Geometry check sheet. Reference: the model listing, model coordinates, mm. Round coordinates to 2 decimals unless told otherwise and drop trailing zeros. Write each loop counter-clockwise with the first axis right and the second up, starting at its lowest first coordinate (ties: lowest second). Pieces come first, ordered by that corner, then holes. Notation, with made-up numbers: (-12.5, -14) - (39.5, -14) arc R28 ccw to (39.5, 15) - close; hole circle Ø8 at (-8.5, -9). An arc over 180 degrees is marked (long way). Return JSON: item names as keys, results as strings. Group by question number.
from build123d import *

# Parameters (mm, degrees)
CROQUIS1_W              = 60
CROQUIS1_H              = 6
SALIENTE_EXTRUIR1_DEPTH = 3
REDONDEO1_R             = 1
CROQUIS2_R              = 1.5
CROQUIS2_R_2            = 1
CORTAR_EXTRUIR1_DEPTH   = 31.298514815


with BuildPart() as part:
    # Croquis1 → Saliente-Extruir1 (new body)
    with BuildSketch(Plane.XY):
        Rectangle(CROQUIS1_W, CROQUIS1_H)
    extrude(amount=SALIENTE_EXTRUIR1_DEPTH)

    # Redondeo1
    redondeo1_edges = [part.edges().sort_by_distance(p)[0] for p in [
        (30, 0, 3),
        (0, 3, 3),
        (-30, 0, 3),
        (0, 3, 0),
        (30, 0, 0),
        (0, -3, 0),
        (-30, 0, 0),
        (0, -3, 3),
    ]]
    fillet(redondeo1_edges, radius=REDONDEO1_R)

    # Croquis2 → Cortar-Extruir1 (cut, through all)
    with BuildSketch(Plane.XY.offset(3)):
        with Locations((-26.35, 0)):
            Circle(CROQUIS2_R)
        with Locations((26.35, 0)):
            Circle(CROQUIS2_R)
        Circle(CROQUIS2_R_2)
    extrude(amount=-CORTAR_EXTRUIR1_DEPTH, mode=Mode.SUBTRACT)


solid = part.part
1. Material ranges on line 1 along Y through (x, z) = (26.35, 1.35); line 2 along X through (y, z) = (1.1, 0.1); line 3 along X through (y, z) = (-0.8, 2.4), recorded low to high.
2. Mould release check, pull along Y, two halves, no side actions. Record for faces 1 (the face through (0, -1, 2)), 2 (the face through (29.715, 0.042, 0.301)), 3 (the face through (24.85, 0.07, 1.52)), 4 (the face through (-0.4, -3, 1.5)): pulls with the +Y half, pulls with the -Y half, needs draft (parallel to the pull), parting line crosses it, or undercut.
3. Depth check by flat-ended pin: pin 1 Ø3 at (x, y) = (0, 0) entering from +Z. Enter the tip coordinate at first touch or a pass-through.
4. Section check C-C (x = 26.35). Enter the section's corners in (y, z), and give its area (3 significant figures).
5. Section check D-D (x = -12). Enter the section's corners in (y, z), and give its area (3 significant figures).
6. Section check A-A (x = 0). Enter the section's corners in (y, z).
7. Section check B-B (y = 0). Enter the section's corners in (x, z).
Result sheet:
{
 "1": {"line 1": "y = -3 to -1.5, 1.5 to 3", "line 2": "x = -29.44 to -27.37, -25.33 to 25.33, 27.37 to 29.44", "line 3": "x = -29.92 to -27.62, -25.08 to -0.6, 0.6 to 25.08, 27.62 to 29.92"},
 "2": {"face 1": "undercut", "face 2": "needs draft", "face 3": "undercut", "face 4": "pulls with the -Y half"},
 "3": {"pin 1": "stops at z = 3"},
 "4": {"outline": "(-3, 1) arc R1 ccw to (-2, 0) - (-1.5, 0) - (-1.5, 3) - (-2, 3) arc R1 ccw to (-3, 2) - close; (1.5, 0) - (2, 0) arc R1 ccw to (3, 1) - (3, 2) arc R1 ccw to (2, 3) - (1.5, 3) - close", "area": "8.14 mm²"},
 "5": {"outline": "(-3, 1) arc R1 ccw to (-2, 0) - (2, 0) arc R1 ccw to (3, 1) - (3, 2) arc R1 ccw to (2, 3) - (-2, 3) arc R1 ccw to (-3, 2) - close", "area": "17.1 mm²"},
 "6": {"outline": "(-3, 1) arc R1 ccw to (-2, 0) - (-1, 0) - (-1, 3) - (-2, 3) arc R1 ccw to (-3, 2) - close; (1, 0) - (2, 0) arc R1 ccw to (3, 1) - (3, 2) arc R1 ccw to (2, 3) - (1, 3) - close"},
 "7": {"outline": "(-30, 1) arc R1 ccw to (-29, 0) - (-27.85, 0) - (-27.85, 3) - (-29, 3) arc R1 ccw to (-30, 2) - close; (-24.85, 0) - (-1, 0) - (-1, 3) - (-24.85, 3) - close; (1, 0) - (24.85, 0) - (24.85, 3) - (1, 3) - close; (27.85, 0) - (29, 0) arc R1 ccw to (30, 1) - (30, 2) arc R1 ccw to (29, 3) - (27.85, 3) - close"}
}
